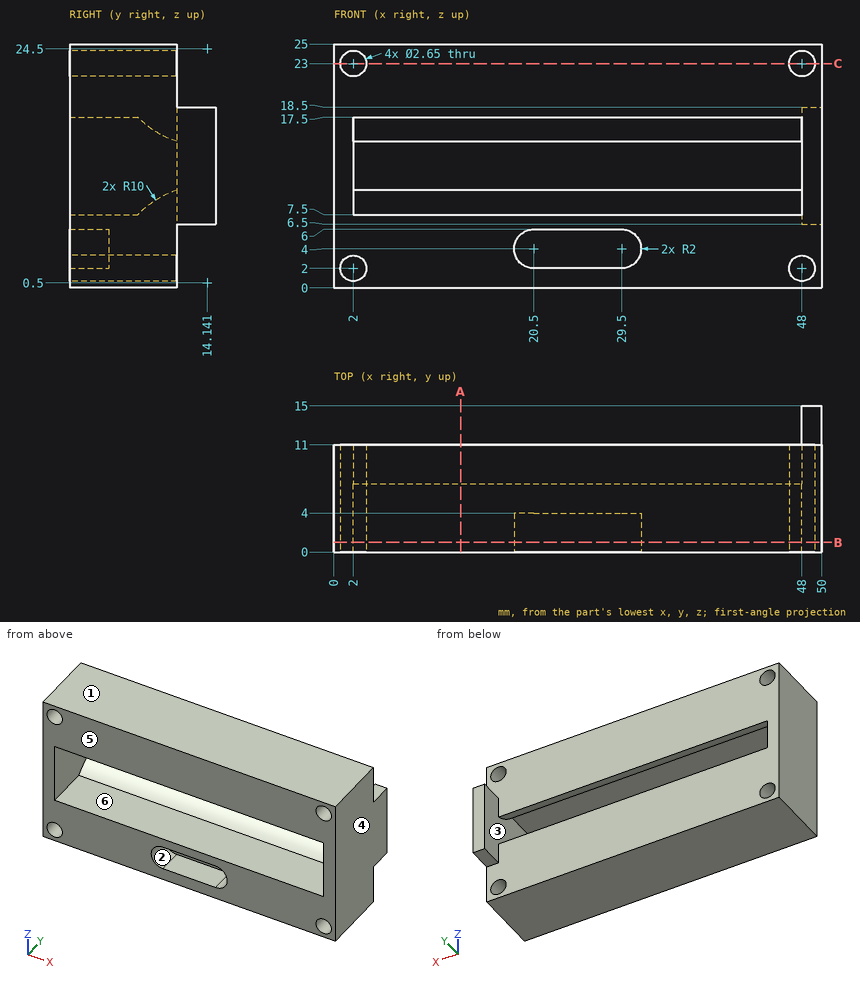
Input: dimensioned drawing with shaded views. Units: mm. Origin: part minimum x, y, z. A direction names the side the tool comes from. Coordinates: 2 decimals unless noted, no trailing zeros. Loops run counter-clockwise (first coordinate to the right, second up) from the corner with the lowest first, then second, coordinate; pieces in that order, holes last. Notation, with made-up numbers: M -11,36.25 L 3,36.25 A7 ccw 3,47.25 Z; hole C -21,35.25 d5. An arc over 180 degrees is marked long. Use a Markdown table: item, result. Add a question column.
1) Section B-B, the plane y = 1. Give the number of separate pieces and of enclosed holes in the cut face.
2) Section A-A, the plane x = 13. Return the cut outline in (y, z).
3) Draft query along X for the marked faces 3, 4, 5 and 6. Return one class per face: +X half, -X half, draft (parallel to the pull), parting line (faces both ways), or undercut.
4) Section C-C, the plane z = 23. Return the cut outline in (x, y) (1 decimal), plus the area to 3 significant figures.
5) Line query: L1, parallel to X at y = 4.5, z = 23 (1 decimal); L2, parallel to X at y = 5, z = 14; L3, parallel to X at y = 11.75, z = 9. Output: solid intervals per line, ascending. Write a range as from..to.
6) Pin query (flat end, axial travel): P1, Ø4, axis at x = 2, z = 2, coming from the -Y side; P2, Ø3, axis at x = 34.5, z = 14, coming from the +Y side; P3, Ø1, axis at x = 6.5, z = 14, coming from the -Y side; P4, Ø1, axis at x = 49, y = 12.5, coming from the -Z side. Return the tip coordinate at first contact, or that it passes through.
7) Set-up query: the marked faces 1 and 2. Return all of +Z, -Z, +X, -X, +Y, -Y with unobstructed straight access to the full face (end or side cutting, diameter ignored); none if empty.
Answer below:
| question | item | result |
|---|---|---|
| 1 | separate pieces | 1 |
| 1 | enclosed holes | 6 |
| 2 | outline | M 0,0 L 11,0 L 11,9.99 A10 ccw 7,7.5 L 0,7.5 Z; M 0,17.5 L 7,17.5 A10 ccw 11,15.01 L 11,25 L 0,25 Z |
| 3 | face 3 | undercut |
| 3 | face 4 | +X half |
| 3 | face 5 | draft |
| 3 | face 6 | undercut |
| 4 | outline | M 0,0 L 0.7,0 L 0.7,11 L 0,11 Z; M 3.3,0 L 46.7,0 L 46.7,11 L 3.3,11 Z; M 49.3,0 L 50,0 L 50,11 L 49.3,11 Z |
| 4 | area | 492 mm2 |
| 5 | L1 | 0..0.7, 3.3..46.7, 49.3..50 |
| 5 | L2 | 0..2, 48..50 |
| 5 | L3 | 48..50 |
| 6 | P1 | y = 0 |
| 6 | P2 | y = 11 |
| 6 | P3 | through |
| 6 | P4 | z = 6.5 |
| 7 | face 1 | +Z, +X, -X, +Y, -Y |
| 7 | face 2 | -Y |
